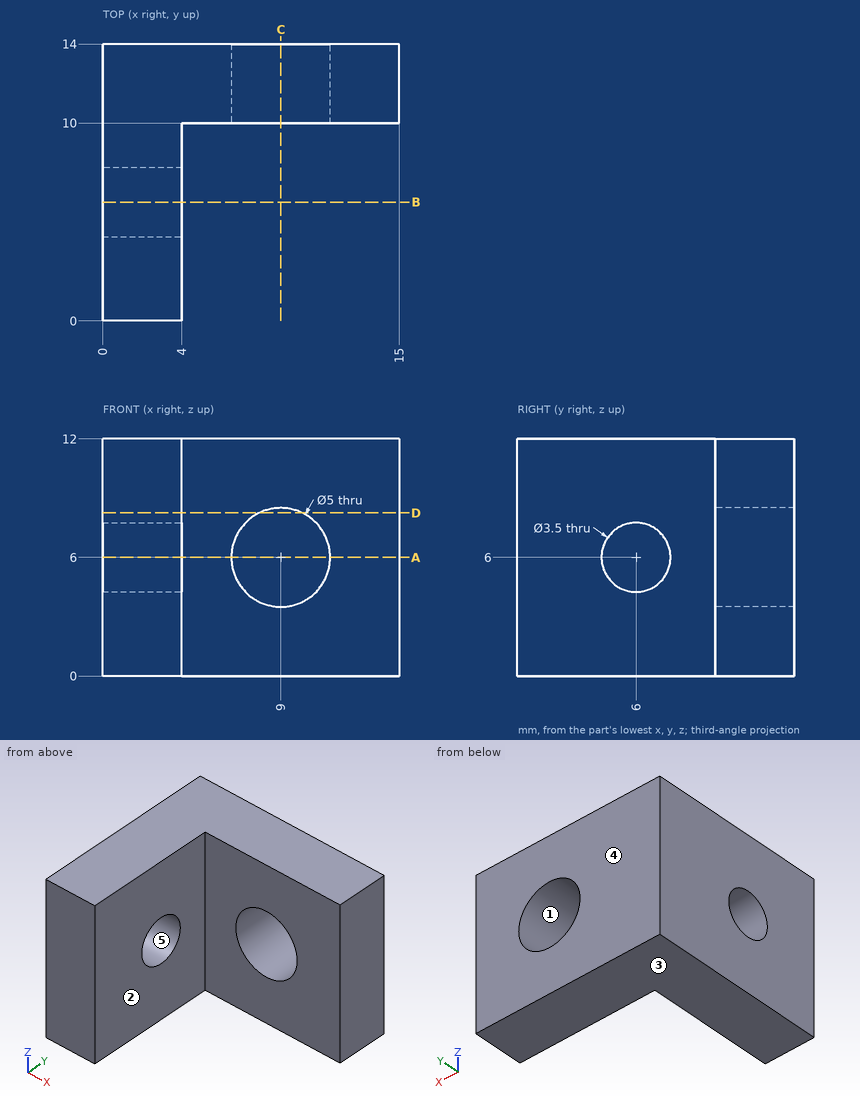
Geometry check sheet. Reference: drawing and pictorial views, mm from the part's lowest x, y, z. A direction names the side the tool comes from. Give positions to 0.01 mm unless a question says otherwise; leave off trailing zeros. Order: outer loops, then holes, each group sorted by start corner. A loop starts at its lowest first (then second) coordinate and runs counter-clockwise, first axis right, second up. Notation, with made-up numbers: (-27.75, 30.25) -> (13.25, 30.25) arc R28 cw to (13.25, 49.25) -> close; hole circle Ø9 at (37, -9.75). An arc over 180 degrees is marked (long way). Use CSV: the item, a comma, the result in double quotes. Start each with the question number.
1) Sectioned sample at C-C, the plane x = 9. Record the boundary of the cut face in (y, z), plus the area to 3 significant figures.
2) Sectioned sample at B-B, the plane y = 6. Record the boundary of the cut face in (x, z), plus the area to 3 significant figures.
3) Mould release check, pull along Y, two halves, no side actions. Record for the marked faces 3, 4 and 5: released by +Y, released by -Y, zero draft, split by the parting line, or undercut.
4) Material ranges on line 1 (Z direction, x = 2.5, y = 6); line 2 (Z direction, x = 9, y = 13.05); line 3 (Y direction, x = 8, z = 0.5), recorded low to high. Write a range as from..to.
5) Go/stop test with a flat-tipped pin: P1, Ø5, axis at y = 5.5, z = 4.5, coming from the +X side. Record where the tip stops, or that it passes through.
6) Sectioned sample at D-D, the plane z = 8.25. Record the boundary of the cut face in (x, y), plus the area to 3 significant figures.
7) Sectioned sample at A-A, the plane z = 6. Record the boundary of the cut face in (x, y), plus the area to 3 significant figures.
8) Set-up check for the marked faces 1 and 2: record each of +Z, -Z, +X, -X, +Y, -Y from which the full face is reachable in a straight line by a thin tool's end or side.
Recorded:
1,outline,"(10, 0) -> (14, 0) -> (14, 3.5) -> (10, 3.5) -> close; (10, 8.5) -> (14, 8.5) -> (14, 12) -> (10, 12) -> close"
1,area,"28.0 mm2"
2,outline,"(0, 0) -> (4, 0) -> (4, 4.25) -> (0, 4.25) -> close; (0, 7.75) -> (4, 7.75) -> (4, 12) -> (0, 12) -> close"
2,area,"34.0 mm2"
3,face 3,"zero draft"
3,face 4,"released by +Y"
3,face 5,"undercut"
4,line 1,"0..4.25, 7.75..12"
4,line 2,"0..3.5, 8.5..12"
4,line 3,"10..14"
5,P1,"x = 4"
6,outline,"(0, 0) -> (4, 0) -> (4, 10) -> (7.91, 10) -> (7.91, 14) -> (0, 14) -> close; (10.09, 10) -> (15, 10) -> (15, 14) -> (10.09, 14) -> close"
6,area,"91.3 mm2"
7,outline,"(0, 0) -> (4, 0) -> (4, 4.25) -> (0, 4.25) -> close; (0, 7.75) -> (4, 7.75) -> (4, 10) -> (6.5, 10) -> (6.5, 14) -> (0, 14) -> close; (11.5, 10) -> (15, 10) -> (15, 14) -> (11.5, 14) -> close"
7,area,"66.0 mm2"
8,face 1,"+Y, -Y"
8,face 2,"+Z, -Z, +X, -Y"
